```python
from build123d import *

# Parameters (mm, degrees)
T_LE_DE_BASE_PLI_E1_DEPTH = 36
TROU_TARAUD_M31_D         = 2.5
D_GAGEMENT_M41_D          = 4.5


# Sheet-metal steps are written as plain solids
with BuildPart() as part:
    # Tôle de base pliée1: sheet metal written as solids
    # Esquisse1 → Tôle de base pliée1 (new body)
    with BuildSketch(Plane(origin=(0, 0, 0), x_dir=(0, 0, -1), z_dir=(1, 0, 0))):
        with BuildLine():
            Line((0, 12.75), (0, 4))
            ThreePointArc((0, 4), (-1.171572875, 1.171572875), (-4, 0))
            Line((-4, 0), (-29, 0))
            Line((-29, 0), (-29, 3))
            Line((-29, 3), (-4, 3))
            ThreePointArc((-4, 3), (-3.292893219, 3.292893219), (-3, 4))
            Line((-3, 4), (-3, 12.75))
            Line((-3, 12.75), (0, 12.75))
        make_face()
    extrude(amount=T_LE_DE_BASE_PLI_E1_DEPTH)

    # Trou taraudé M31 (through all)
    with Locations(Plane(origin=(0, 3, 0), x_dir=(1, 0, 0), z_dir=(0, 1, 0))):
        with Locations((4.5, -24.5), (4.5, -8.5), (20.5, -8.5), (20.5, -24.5)):
            Hole(TROU_TARAUD_M31_D / 2)

    # Dégagement M41 (through all)
    with Locations(Plane.XY.offset(3)):
        with Locations((18, 8.2)):
            Hole(D_GAGEMENT_M41_D / 2)


solid = part.part
```
Work out the finished part from the listing and answer in its coordinate system (mm). A direction names the side the tool comes from. Round coordinates to 2 decimals unless told otherwise and drop trailing zeros. Write each loop counter-clockwise with the first axis right and the second up, starting at its lowest first coordinate (ties: lowest second). Pieces come first, ordered by that corner, then holes. Notation, with made-up numbers: (-15.75, 46.5) -> (38.25, 46.5) arc R7 ccw to (38.25, 59.5) -> close; hole circle Ø6 at (86, -22.75). An arc over 180 degrees is marked (long way). Write each question's results on one line, items separated by ' | '.
Q1. Which of the six approach directions +Z, -Z, +X, -X, +Y, -Y give full straight-line access (tool end or side, diameter ignored) to faces 1 (the cylindrical face through (16.962, 6.204, 1.479)), 2 (the flat face through (18, 11, 3))?
Data:
face 1: +Z, -Z | face 2: +Z, +X, -X, +Y
Q2. Flat-ended cylindrical pins translate along their axes: P1, Ø3, axis at x = 4.5, z = 8.5, coming from the +Y side; P2, Ø6, axis at x = 13, z = 14.5, coming from the -Y side. Find the tip coordinate at first contact, or state that the pin passes through.
Data:
P1: y = 3 | P2: y = 0
Q3. Section A-A, the plane y = 8.2 is taken. Write down the section's boundary in (x, z).
Data:
outline: (0, 0) -> (15.75, 0) -> (15.75, 3) -> (0, 3) -> close; (20.25, 0) -> (36, 0) -> (36, 3) -> (20.25, 3) -> close
Q4. Determine the mould class of faces 3 (the cylindrical face through (4.77, 1.48, 9.72)), 4 (the flat face through (36, 2.6, 11.2)), 5 (the flat face through (18, 1, 29)) for opening direction X: released by +X, released by -X, zero draft, split by the parting line, or undercut.
Data:
face 3: undercut | face 4: released by +X | face 5: zero draft
Q5. Section C-C, the plane z = 8.5 is taken. Write down the section's boundary in (x, y).
Data:
outline: (0, 0) -> (3.25, 0) -> (3.25, 3) -> (0, 3) -> close; (5.75, 0) -> (19.25, 0) -> (19.25, 3) -> (5.75, 3) -> close; (21.75, 0) -> (36, 0) -> (36, 3) -> (21.75, 3) -> close
Q6. Section D-D, the plane x = 4.5 is taken. Write down the section's boundary in (y, z).
Data:
outline: (0, 4) arc R4 ccw to (4, 0) -> (12.75, 0) -> (12.75, 3) -> (4, 3) arc R1 cw to (3, 4) -> (3, 7.25) -> (0, 7.25) -> close; (0, 9.75) -> (3, 9.75) -> (3, 23.25) -> (0, 23.25) -> close; (0, 25.75) -> (3, 25.75) -> (3, 29) -> (0, 29) -> close
Q7. Section B-B, the plane x = 18 is taken. Write down the section's boundary in (y, z).
Data:
outline: (0, 4) arc R4 ccw to (4, 0) -> (5.95, 0) -> (5.95, 3) -> (4, 3) arc R1 cw to (3, 4) -> (3, 29) -> (0, 29) -> close; (10.45, 0) -> (12.75, 0) -> (12.75, 3) -> (10.45, 3) -> close
Q8. Straight lines are drawn through the part: line 1 along X through (y, z) = (0.6, 8.5); line 2 along Z through (x, y) = (4.5, 2); line 3 along Z through (x, y) = (20.5, 1.15). For each, find the intervals that lie inside material, in ascending order. Write a range as [from, to].
Data:
line 1: [0, 3.25], [5.75, 19.25], [21.75, 36] | line 2: [0.54, 7.25], [9.75, 23.25], [25.75, 29] | line 3: [1.19, 7.25], [9.75, 23.25], [25.75, 29]
